from build123d import *

# Parameters (mm, degrees)
SKETCH1_R           = 70
SKETCH1_R_2         = 3.3
SKETCH1_R_3         = 3
BOSS_EXTRUDE1_DEPTH = 7.5


with BuildPart() as part:
    # Sketch1 → Boss-Extrude1 (new, symmetric)
    with BuildSketch(Plane.XY):
        Circle(SKETCH1_R)
        with Locations((64, 0)):
            Circle(SKETCH1_R_2, mode=Mode.SUBTRACT)
        with Locations((45.254833996, 45.254833996)):
            Circle(SKETCH1_R_2, mode=Mode.SUBTRACT)
        with Locations((0, 64)):
            Circle(SKETCH1_R_2, mode=Mode.SUBTRACT)
        with Locations((-45.254833996, 45.254833996)):
            Circle(SKETCH1_R_2, mode=Mode.SUBTRACT)
        with Locations((-64, 0)):
            Circle(SKETCH1_R_2, mode=Mode.SUBTRACT)
        with Locations((-45.254833996, -45.254833996)):
            Circle(SKETCH1_R_2, mode=Mode.SUBTRACT)
        with Locations((0, -64)):
            Circle(SKETCH1_R_2, mode=Mode.SUBTRACT)
        with Locations((45.254833996, -45.254833996)):
            Circle(SKETCH1_R_2, mode=Mode.SUBTRACT)
        with Locations((24.491739671, 59.128290081)):
            Circle(SKETCH1_R_3, mode=Mode.SUBTRACT)
        with Locations((-24.491739671, -59.128290081)):
            Circle(SKETCH1_R_3, mode=Mode.SUBTRACT)
        with BuildLine():
            Line((2.437233269, 55.821819381), (-2.437233269, 55.821819381))
            ThreePointArc((-2.437233269, 55.821819381), (-48.389169436, 27.9375), (-49.561730304, -25.800203765))
            Line((-49.561730304, -25.800203765), (-47.124497035, -30.021615616))
            ThreePointArc((-47.124497035, -30.021615616), (0, -55.875), (47.124497035, -30.021615616))
            Line((47.124497035, -30.021615616), (49.561730304, -25.800203765))
            ThreePointArc((49.561730304, -25.800203765), (48.389169436, 27.9375), (2.437233269, 55.821819381))
        make_face(mode=Mode.SUBTRACT)
    extrude(amount=BOSS_EXTRUDE1_DEPTH, both=True)


solid = part.part
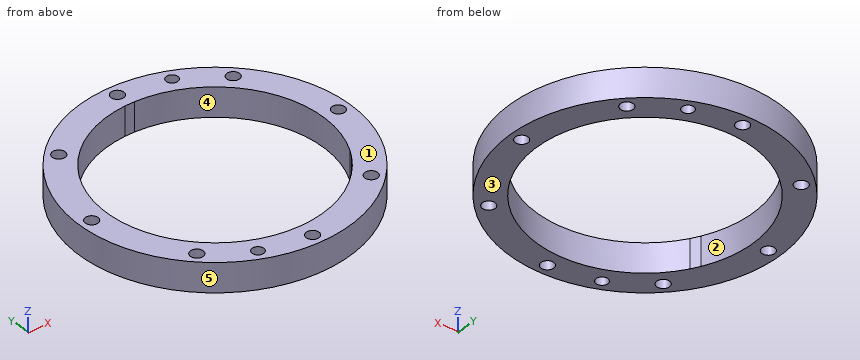
Geometry check sheet. Reference: the model listing, model coordinates, mm. Face numbers are marked on the shaded views. A direction names the side the tool comes from. Round coordinates to 2 decimals unless told otherwise and drop trailing zeros. Loops run counter-clockwise (first coordinate to the right, second up) from the corner with the lowest first, then second, coordinate; pieces in that order, holes last. Notation, with made-up numbers: (-26, 5) - (-1, 5) arc R16 ccw to (-1, 21) - close; hole circle Ø9 at (22, 46.25). An arc over 180 degrees is marked (long way). One line per question, with ' | ' between items. Start each with the question number.
1. Cross-section at A-A on x = 0. Record the cut outline in (y, z) (3 decimals), then the cut area to 3 significant figures.
2. Cross-section at D-D on y = 24.5. Record the cut outline in (x, z), then the cut area to 3 significant figures.
3. Scan lines: line 1 (Y direction, x = 0, z = 2) (3 decimals); line 2 (X direction, y = 42.5, z = -0.5); line 3 (X direction, y = -18.5, z = -3.75). Record each from-to range of solid material in increasing order. Write a range as [from, to].
4. Cross-section at B-B on y = 0. Record the cut outline in (x, z) (3 decimals).
5. Depth check by flat-ended pin: pin 1 (1 mm diameter, centred on x = 53.5, z = 4, fed in from +Y); pin 2 (4 mm diameter, centred on y = -53.5, z = -1, fed in from -X); pin 3 (5 mm diameter, centred on y = -48, z = -3.5, fed in from -X). Enter the tip coordinate at first touch or a pass-through.
6. Tool access check on the marked faces 1 and 2. Record the directions out of +Z, -Z, +X, -X, +Y, -Y that give a thin tool (end or side, any length) a straight path to the whole face; none if there is none.
7. Cross-section at C-C on z = -1.5. State how many separate pieces and enclosed holes the cut face has, then the cut area to 3 significant figures.
8. Draft check along X on the marked faces 3, 4 and 5. Enter one of: released by +X, released by -X, zero draft, split by the parting line, or undercut.
Taken from the geometry:
1) outline: (-70, -7.5) - (-67.3, -7.5) - (-67.3, 7.5) - (-70, 7.5) - close; (-60.7, -7.5) - (-55.875, -7.5) - (-55.875, 7.5) - (-60.7, 7.5) - close; (55.822, -7.5) - (60.7, -7.5) - (60.7, 7.5) - (55.822, 7.5) - close; (67.3, -7.5) - (70, -7.5) - (70, 7.5) - (67.3, 7.5) - close | area: 227 mm²
2) outline: (-65.57, -7.5) - (-50.22, -7.5) - (-50.22, 7.5) - (-65.57, 7.5) - close; (50.22, -7.5) - (65.57, -7.5) - (65.57, 7.5) - (50.22, 7.5) - close | area: 461 mm²
3) line 1: [-70, -67.3], [-60.7, -55.875], [55.822, 60.7], [67.3, 70] | line 2: [-55.62, -47.07], [-43.44, -36.27], [36.27, 43.44], [47.07, 55.62] | line 3: [-67.51, -52.72], [52.72, 67.51]
4) outline: (-70, -7.5) - (-67.3, -7.5) - (-67.3, 7.5) - (-70, 7.5) - close; (-60.7, -7.5) - (-55.875, -7.5) - (-55.875, 7.5) - (-60.7, 7.5) - close; (55.875, -7.5) - (60.7, -7.5) - (60.7, 7.5) - (55.875, 7.5) - close; (67.3, -7.5) - (70, -7.5) - (70, 7.5) - (67.3, 7.5) - close
5) pin 1: y = 45.73 | pin 2: x = -47.41 | pin 3: x = -53.2
6) face 1: +Z, +X, -X, +Y, -Y | face 2: +Z, -Z
7) separate pieces: 1 | enclosed holes: 11 | area: 5,260 mm²
8) face 3: zero draft | face 4: undercut | face 5: split by the parting line
